```python
from build123d import *

# Parameters (mm, degrees)
PAD002_DEPTH        = 25
THICKNESS_T         = -2.5
SKETCH003_W         = 33
SKETCH003_H         = 18
POCKET_DEPTH        = 5
CHAMFER_SIZE        = 2
SKETCH004_W         = 19
SKETCH004_H         = 12.5
POCKET001_DEPTH     = 5
SKETCH005_R         = 2
POCKET002_DEPTH     = 5
SKETCH006_W         = 11.5
SKETCH006_H         = 4
POCKET003_DEPTH     = 5
SKETCH007_R         = 8.75
POCKET004_DEPTH     = 1
SKETCH011_W         = 40
SKETCH011_H         = 16
POCKET005_DEPTH     = 38.501
SKETCH012_W         = 16
SKETCH012_H         = 40
PAD005_DEPTH        = 2.5
SKETCH013_W         = 16
SKETCH013_H         = 13.5
PAD006_DEPTH        = 2.5
PAD007_DEPTH        = 2.5
SKETCH014_W         = 11
SKETCH014_H         = 6
POCKET006_DEPTH     = 2.5
SKETCH015_W         = 11
SKETCH015_H         = 2.5
PAD008_DEPTH        = 6
SKETCH016_R         = 2.5
PAD009_DEPTH        = 22.5
SKETCH017_R         = 0.75
POCKET007_DEPTH     = 18
SKETCH018_R         = 2.5
SKETCH018_R_2       = 0.75
PAD010_DEPTH        = 9
FILLET001_R         = 3
FILLET002_R         = 3
FILLET003_R         = 3
FILLET005_R         = 2
SKETCH020_R         = 1.45
POCKET009_DEPTH     = 5
FILLET006_R         = 2
FILLET006_FACE100_W = 11
FILLET006_FACE100_H = 6
PAD011_DEPTH        = 4
PAD011_FACE78_R     = 8.75
PAD011_FACE78_R_2   = 1.45
PAD012_DEPTH        = 1
SKETCH021_R         = 9
POCKET010_DEPTH     = 1


with BuildPart() as part:
    # Sketch002 → Pad002 (new body)
    with BuildSketch(Plane.XY):
        Polygon((-10, 80), (-71, 80), (-71, 0), (-48.5, 0), (-48.5, -40), (-32.5, -40), (-32.5, 0), (-10, 0), align=None)
    extrude(amount=PAD002_DEPTH)

    # Thickness
    thickness_openings = [part.faces().sort_by_distance(p)[0] for p in [
        (-40.5, 33.043478, 25),
    ]]
    offset(amount=THICKNESS_T, openings=thickness_openings)

    # Sketch003 (on Face9 of Thickness) → Pocket (cut)
    with BuildSketch(Plane(origin=(0, 0, 0), x_dir=(1, 0, 0), z_dir=(0, 0, -1))):
        with Locations((-40.5, -61)):
            Rectangle(SKETCH003_W, SKETCH003_H)
    extrude(amount=-POCKET_DEPTH, mode=Mode.SUBTRACT)

    # Chamfer
    chamfer_edges = [part.edges().sort_by_distance(p)[0] for p in [
        (-40.5, 70, 0),
        (-57, 61, 0),
        (-40.5, 52, 0),
        (-24, 61, 0),
    ]]
    chamfer(chamfer_edges, length=CHAMFER_SIZE)

    # Sketch004 (on Face1 of Chamfer) → Pocket001 (cut)
    with BuildSketch(Plane(origin=(0, 0, 0), x_dir=(1, 0, 0), z_dir=(0, 0, -1))):
        with Locations((-29.5, -11.25)):
            Rectangle(SKETCH004_W, SKETCH004_H)
    extrude(amount=-POCKET001_DEPTH, mode=Mode.SUBTRACT)

    # Sketch005 (on Face1 of Pocket001) → Pocket002 (cut)
    with BuildSketch(Plane(origin=(0, 0, 0), x_dir=(1, 0, 0), z_dir=(0, 0, -1))):
        with Locations((-56, -12)):
            Circle(SKETCH005_R)
    extrude(amount=-POCKET002_DEPTH, mode=Mode.SUBTRACT)

    # Sketch006 (on Face26 of Pocket002) → Pocket003 (cut)
    with BuildSketch(Plane.XZ.offset(-77.5)):
        with Locations((-54.75, 19)):
            Rectangle(SKETCH006_W, SKETCH006_H)
    extrude(amount=-POCKET003_DEPTH, mode=Mode.SUBTRACT)

    # Sketch007 (on Face1 of Pocket003) → Pocket004 (cut)
    with BuildSketch(Plane(origin=(0, 0, 0), x_dir=(1, 0, 0), z_dir=(0, 0, -1))):
        with Locations((-56, -33)):
            Circle(SKETCH007_R)
    extrude(amount=-POCKET004_DEPTH, mode=Mode.SUBTRACT)

    # Sketch011 (on Face8 of Pocket004) → Pocket005 (cut, through all)
    with BuildSketch(Plane(origin=(-48.5, 0, 0), x_dir=(0, -1, 0), z_dir=(-1, 0, 0))):
        with Locations((20, 8)):
            Rectangle(SKETCH011_W, SKETCH011_H)
    extrude(amount=-POCKET005_DEPTH, mode=Mode.SUBTRACT)

    # Sketch012 (on Face20 of Pocket005) → Pad005 (join)
    with BuildSketch(Plane(origin=(0, 0, 16), x_dir=(1, 0, 0), z_dir=(0, 0, -1))):
        with Locations((-40.5, 20)):
            Rectangle(SKETCH012_W, SKETCH012_H)
    extrude(amount=PAD005_DEPTH)

    # Sketch013 (on Face4 of Pad005) → Pad006 (join)
    with BuildSketch(Plane.XZ):
        with Locations((-40.5, 6.75)):
            Rectangle(SKETCH013_W, SKETCH013_H)
    extrude(amount=-PAD006_DEPTH)

    # Pad006 Face50 → Pad007 (add)
    with BuildSketch(Plane(origin=(-40.5, 1.311465, 13.5), x_dir=(0, 1, 0), z_dir=(0, 0, 1))):
        with BuildLine():
            ThreePointArc((1.188535, 8), (0.456302, 6.232233), (-1.311465, 5.5))
            Line((-1.311465, 5.5), (-1.311465, -5.5))
            ThreePointArc((-1.311465, -5.5), (0.456302, -6.232233), (1.188535, -8))
            Line((1.188535, -8), (1.188535, 8))
        make_face()
    extrude(amount=PAD007_DEPTH)

    # Sketch014 (on Face35 of Pad007) → Pocket006 (cut)
    with BuildSketch(Plane(origin=(0, 0, 13.5), x_dir=(1, 0, 0), z_dir=(0, 0, -1))):
        with Locations((-40.5, 34.5)):
            Rectangle(SKETCH014_W, SKETCH014_H)
    extrude(amount=-POCKET006_DEPTH, mode=Mode.SUBTRACT)

    # Sketch015 (on Face56 of Pocket006) → Pad008 (join)
    with BuildSketch(Plane.XY.offset(16)):
        with Locations((-40.5, -30.25)):
            Rectangle(SKETCH015_W, SKETCH015_H)
    extrude(amount=PAD008_DEPTH)

    # Sketch016 (on Face28 of Pad008) → Pad009 (join)
    with BuildSketch(Plane.XY.offset(2.5)):
        with Locations((-66.5, 75.5)):
            Circle(SKETCH016_R)
        with Locations((-14.5, 75.5)):
            Circle(SKETCH016_R)
        with Locations((-66.5, 4.5)):
            Circle(SKETCH016_R)
        with Locations((-14.5, 4.5)):
            Circle(SKETCH016_R)
    extrude(amount=PAD009_DEPTH)

    # Sketch017 (on Face79 of Pad009) → Pocket007 (cut)
    with BuildSketch(Plane.XY.offset(25)):
        with Locations((-66.5, 4.5)):
            Circle(SKETCH017_R)
        with Locations((-14.5, 4.5)):
            Circle(SKETCH017_R)
        with Locations((-14.5, 75.5)):
            Circle(SKETCH017_R)
        with Locations((-66.5, 75.5)):
            Circle(SKETCH017_R)
    extrude(amount=-POCKET007_DEPTH, mode=Mode.SUBTRACT)

    # Sketch018 (on Face84 of Pocket007) → Pad010 (join)
    with BuildSketch(Plane.XY.offset(16)):
        with Locations((-40.5, -24)):
            Circle(SKETCH018_R)
        with Locations((-40.5, -24)):
            Circle(SKETCH018_R_2, mode=Mode.SUBTRACT)
    extrude(amount=PAD010_DEPTH)

    # Fillet001
    fillet001_edges = [part.edges().sort_by_distance(p)[0] for p in [
        (-71, 80, 12.5),
    ]]
    fillet(fillet001_edges, radius=FILLET001_R)

    # Fillet002
    fillet002_edges = [part.edges().sort_by_distance(p)[0] for p in [
        (-10, 80, 12.5),
    ]]
    fillet(fillet002_edges, radius=FILLET002_R)

    # Fillet003
    fillet003_edges = [part.edges().sort_by_distance(p)[0] for p in [
        (-10, 0, 8),
        (-10, 0, 20.5),
        (-71, 0, 12.5),
    ]]
    fillet(fillet003_edges, radius=FILLET003_R)

    # Fillet005
    fillet005_edges = [part.edges().sort_by_distance(p)[0] for p in [
        (-32.5, -20, 13.5),
        (-48.5, -20, 13.5),
    ]]
    fillet(fillet005_edges, radius=FILLET005_R)

    # Sketch020 (on Face71 of Fillet005) → Pocket009 (cut)
    with BuildSketch(Plane(origin=(0, 0, 1), x_dir=(1, 0, 0), z_dir=(0, 0, -1))):
        with Locations((-58.774455, -26.301873)):
            Circle(SKETCH020_R)
        with Locations((-53.225545, -26.301873)):
            Circle(SKETCH020_R)
        with Locations((-49.954328, -37.001543)):
            Circle(SKETCH020_R)
        with Locations((-61.081592, -38.171066)):
            Circle(SKETCH020_R)
    extrude(amount=-POCKET009_DEPTH, mode=Mode.SUBTRACT)

    # Fillet006
    fillet006_edges = [part.edges().sort_by_distance(p)[0] for p in [
        (-22.75, 0, 0),
    ]]
    fillet(fillet006_edges, radius=FILLET006_R)

    # Fillet006 Face100 → Pad011 (add)
    with BuildSketch(Plane(origin=(-40.5, -29, 19), x_dir=(1, 0, 0), z_dir=(0, 1, 0))):
        Rectangle(FILLET006_FACE100_W, FILLET006_FACE100_H)
    extrude(amount=PAD011_DEPTH)

    # Pad011 Face78 → Pad012 (add)
    with BuildSketch(Plane(origin=(-56.029742, 33.130299, 1), x_dir=(0, -1, 0), z_dir=(0, 0, -1))):
        with Locations((0.130299, -0.029742)):
            Circle(PAD011_FACE78_R)
        with Locations((6.828426, 2.744713)):
            Circle(PAD011_FACE78_R_2, mode=Mode.SUBTRACT)
        with Locations((6.828426, -2.804197)):
            Circle(PAD011_FACE78_R_2, mode=Mode.SUBTRACT)
        with Locations((-5.040767, 5.05185)):
            Circle(PAD011_FACE78_R_2, mode=Mode.SUBTRACT)
        with Locations((-3.871244, -6.075414)):
            Circle(PAD011_FACE78_R_2, mode=Mode.SUBTRACT)
    extrude(amount=PAD012_DEPTH)

    # Sketch021 (on Face77 of Pad012) → Pocket010 (cut)
    with BuildSketch(Plane.XY.offset(2.5)):
        with Locations((-56, 33)):
            Circle(SKETCH021_R)
    extrude(amount=-POCKET010_DEPTH, mode=Mode.SUBTRACT)


solid = part.part
```
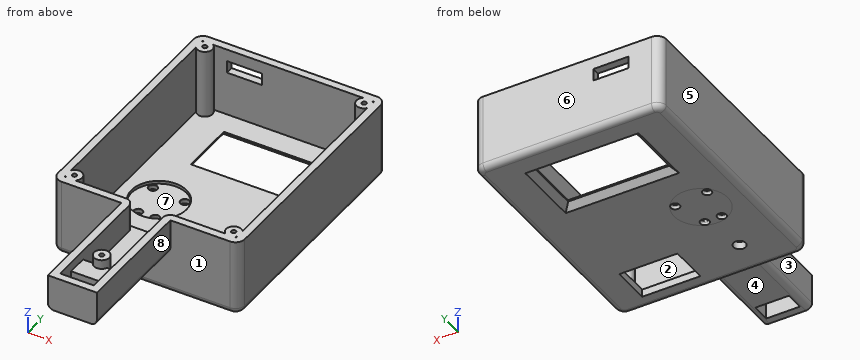
Can you work these out from the model? Positions are in its coordinate system, mm. Face numbers are marked on the shaded views. A direction names the side the tool comes from. Coordinates: 2 decimals unless noted, no trailing zeros. Loops run counter-clockwise (first coordinate to the right, second up) from the corner with the lowest first, then second, coordinate; pieces in that order, holes last. Notation, with made-up numbers: (-34.75, 66) -> (22.25, 66) arc R13 cw to (22.25, 75) -> close; hole circle Ø11 at (71.25, 38). An arc over 180 degrees is marked (long way). Answer as a JSON object with one key per item and string values.
1) Thinking about a two-plate mould opening in X: for the marked faces 5, 6, 7 and 8, which applies, pulls with the +X half, pulls with the -X half, needs draft (parallel to the pull), parting line crosses it, or undercut?
Results:
{"face 5": "pulls with the -X half", "face 6": "needs draft", "face 7": "undercut", "face 8": "pulls with the +X half"}
2) For P1, Ø1.2, axis at y = 79, z = 20, coming from the +X side; P2, Ø1.6, axis at x = -14.5, y = 4.5, coming from the +Z side; P3, Ø3, axis at y = -19.5, z = 21, coming from the -X side; P4, Ø1, axis at x = -58, y = 40, coming from the +Z side, each with a flat end and sliding along its axis, tell me the tip position at first contact or that it passes through.
Results:
{"P1": "stops at x = -10.35", "P2": "stops at z = 25", "P3": "stops at x = -48.5", "P4": "stops at z = 1.5"}
3) Imagine slicing it at C-C (z = 11.75). Count the separate pieces of the cut face and the enclosed holes in it, then the cut area to 3 significant figures.
Results:
{"separate pieces": "1", "enclosed holes": "9", "area": "736 mm^2"}
4) For the marked faces 1, 2, 3 and 4, which set-ups out of +Z, -Z, +X, -X, +Y, -Y let a thin tool reach every point of the face, with its end or its side?
Results:
{"face 1": "-Z, -Y", "face 2": "+Z", "face 3": "+Z, -Z, -X, -Y", "face 4": "-Z, +X, -X, -Y"}
5) If I drill on line 1 (Y direction, x = -56, z = 2.35); line 2 (Y direction, x = -14.5, z = 17); line 3 (X direction, y = 12, z = 23.5), over which ranges is the centre line in solid material (lowest first)?
Results:
{"line 1": "y = 0 to 10, 14 to 24, 42 to 52, 70 to 80", "line 2": "y = 0 to 3.75, 5.25 to 7, 73 to 74.75, 76.25 to 80", "line 3": "x = -71 to -68.5, -12.5 to -10"}
6) Imagine slicing it at A-A (y = 12). Please give me the cut outline in (x, z), then the cut area to 3 significant figures.
Results:
{"outline": "(-71, 2) arc R2 ccw to (-69, 0) -> (-58, 0) -> (-58, 2.5) -> (-68.5, 2.5) -> (-68.5, 25) -> (-71, 25) -> close; (-54, 0) -> (-39, 0) -> (-39, 2.5) -> (-54, 2.5) -> close; (-20, 0) -> (-12, 0) arc R2 ccw to (-10, 2) -> (-10, 25) -> (-12.5, 25) -> (-12.5, 2.5) -> (-20, 2.5) -> close", "area": "206 mm^2"}
7) Imagine slicing it at B-B (x = -18.5). Please give me the cut outline in (y, z).
Results:
{"outline": "(0, 2) arc R2 ccw to (2, 0) -> (78, 0) arc R2 ccw to (80, 2) -> (80, 25) -> (77.5, 25) -> (77.5, 2.5) -> (2.5, 2.5) -> (2.5, 25) -> (0, 25) -> close"}
8) Imagine slicing it at D-D (y = -17). Please give me the cut outline in (x, z).
Results:
{"outline": "(-48.5, 15.5) arc R2 ccw to (-46.5, 13.5) -> (-34.5, 13.5) arc R2 ccw to (-32.5, 15.5) -> (-32.5, 25) -> (-35, 25) -> (-35, 16) -> (-46, 16) -> (-46, 25) -> (-48.5, 25) -> close"}
